from build123d import *

# Parameters (mm, degrees)
SKETCH_1_W          = 30
SKETCH_1_H          = 766.14
SKETCH_1_R          = 2
SKETCH_1_R_2        = 1.999999998
EXTRUDE_2_DEPTH     = 70
SKETCH_2_W          = 26
SKETCH_2_H          = 66
CUT_EXTRUDE_3_DEPTH = 767.14
SKETCH_3_W          = 30
SKETCH_3_H          = 624.936750841
CUT_EXTRUDE_4_DEPTH = 71
SKETCH_4_R          = 3
CUT_EXTRUDE_5_DEPTH = 115


with BuildPart() as part:
    # 草图1 → 凸台-拉伸2 (new body)
    with BuildSketch(Plane.XY):
        Rectangle(SKETCH_1_W, SKETCH_1_H)
        with Locations((-7.500000035, 377.074776011)):
            Circle(SKETCH_1_R, mode=Mode.SUBTRACT)
        with Locations((7.499999965, 377.074776011)):
            Circle(SKETCH_1_R, mode=Mode.SUBTRACT)
        with Locations((-7.500000035, 352.074776011)):
            Circle(SKETCH_1_R, mode=Mode.SUBTRACT)
        with Locations((7.499999965, 352.074776011)):
            Circle(SKETCH_1_R, mode=Mode.SUBTRACT)
        with Locations((7.499878903, 260.000000008)):
            Circle(SKETCH_1_R_2, mode=Mode.SUBTRACT)
        with Locations((-7.500121097, 260.000000008)):
            Circle(SKETCH_1_R_2, mode=Mode.SUBTRACT)
    extrude(amount=EXTRUDE_2_DEPTH)

    # 草图2 → 切除-拉伸3 (cut, through all)
    with BuildSketch(Plane.XZ.offset(383.07)):
        with Locations((0, 35)):
            Rectangle(SKETCH_2_W, SKETCH_2_H)
    extrude(amount=-CUT_EXTRUDE_3_DEPTH, mode=Mode.SUBTRACT)

    # 草图3 → 切除-拉伸4 (cut, through all)
    with BuildSketch(Plane.XY.offset(70)):
        with Locations((0, -82.468375421)):
            Rectangle(SKETCH_3_W, SKETCH_3_H)
    extrude(amount=-CUT_EXTRUDE_4_DEPTH, mode=Mode.SUBTRACT)

    # 草图4 → 切除-拉伸5 (cut)
    with BuildSketch(Plane.XY.offset(70)):
        with Locations((-7.500000035, 377.074776011)):
            Circle(SKETCH_4_R)
        with Locations((7.499999965, 377.074776011)):
            Circle(SKETCH_4_R)
        with Locations((7.499999965, 352.074776011)):
            Circle(SKETCH_4_R)
        with Locations((-7.500000035, 352.074776011)):
            Circle(SKETCH_4_R)
        with Locations((-7.500121097, 260.000000008)):
            Circle(SKETCH_4_R)
        with Locations((7.499878903, 260.000000008)):
            Circle(SKETCH_4_R)
    extrude(amount=-CUT_EXTRUDE_5_DEPTH, mode=Mode.SUBTRACT)


solid = part.part
Input: part model. Units: mm. Frame: model coordinates. A direction names the side the tool comes from. Give positions to 0.01 mm unless a question says otherwise; leave off trailing zeros. Write each loop counter-clockwise with the first axis right and the second up, starting at its lowest first coordinate (ties: lowest second). Pieces come first, ordered by that corner, then holes.
Q1. Section B-B, the plane z = 28.5. Output: boundary loops of the cut face in (x, y), plus the area to 3 significant figures.
Q2. Pull-direction query (X, two-part tool) for faces 3 (the face through (-13.4, 230, 37.8)), 4 (the face through (7.109, 262.974, 1.014)), 5 (the face through (-7.891, 262.974, 1.014)), 6 (the face through (-15, 305, 35)); classes: pulls with the +X half, pulls with the -X half, needs draft (parallel to the pull), parting line crosses it, or undercut.
Q3. Section D-D, the plane y = 339. Output: boundary loops of the cut face in (x, z), plus the area to 3 significant figures.
Q4. Material intervals for probe 1 along Y at (x, z) = (7.5, 69.2); probe 2 along X at (y, z) = (251, 56.5); probe 3 along Z at (x, y) = (11, 315), sorted ascending.
Q5. Section A-A, the plane y = 260. Output: boundary loops of the cut face in (x, z), plus the area to 3 significant figures.
Q6. Set-up query: faces 1 (the face through (-7.891, 262.974, 69.014)), 2 (the face through (13, 305, 35)). Return all of +Z, -Z, +X, -X, +Y, -Y with unobstructed straight access to the full face (end or side cutting, diameter ignored); none if empty.
Q7. Section C-C, the plane x = 2. Output: boundary loops of the cut face in (y, z).
Filled in:
1. outline: (-15, 230) - (-13, 230) - (-13, 383.07) - (-15, 383.07) - close; (13, 230) - (15, 230) - (15, 383.07) - (13, 383.07) - close
1. area: 612 mm2
2. face 3: needs draft
2. face 4: undercut
2. face 5: undercut
2. face 6: pulls with the -X half
3. outline: (-15, 0) - (15, 0) - (15, 70) - (-15, 70) - close; hole (-13, 2) - (13, 2) - (13, 68) - (-13, 68) - close
3. area: 384 mm2
4. probe 1: y = 230 to 257, 263 to 349.07, 355.07 to 374.07, 380.07 to 383.07
4. probe 2: x = -15 to -13, 13 to 15
4. probe 3: z = 0 to 2, 68 to 70
5. outline: (-15, 0) - (-10.5, 0) - (-10.5, 2) - (-13, 2) - (-13, 68) - (-10.5, 68) - (-10.5, 70) - (-15, 70) - close; (-4.5, 0) - (4.5, 0) - (4.5, 2) - (-4.5, 2) - close; (-4.5, 68) - (4.5, 68) - (4.5, 70) - (-4.5, 70) - close; (10.5, 0) - (15, 0) - (15, 70) - (10.5, 70) - (10.5, 68) - (13, 68) - (13, 2) - (10.5, 2) - close
5. area: 336 mm2
6. face 1: +Z, -Z
6. face 2: +Y, -Y
7. outline: (230, 0) - (383.07, 0) - (383.07, 2) - (230, 2) - close; (230, 68) - (383.07, 68) - (383.07, 70) - (230, 70) - close
